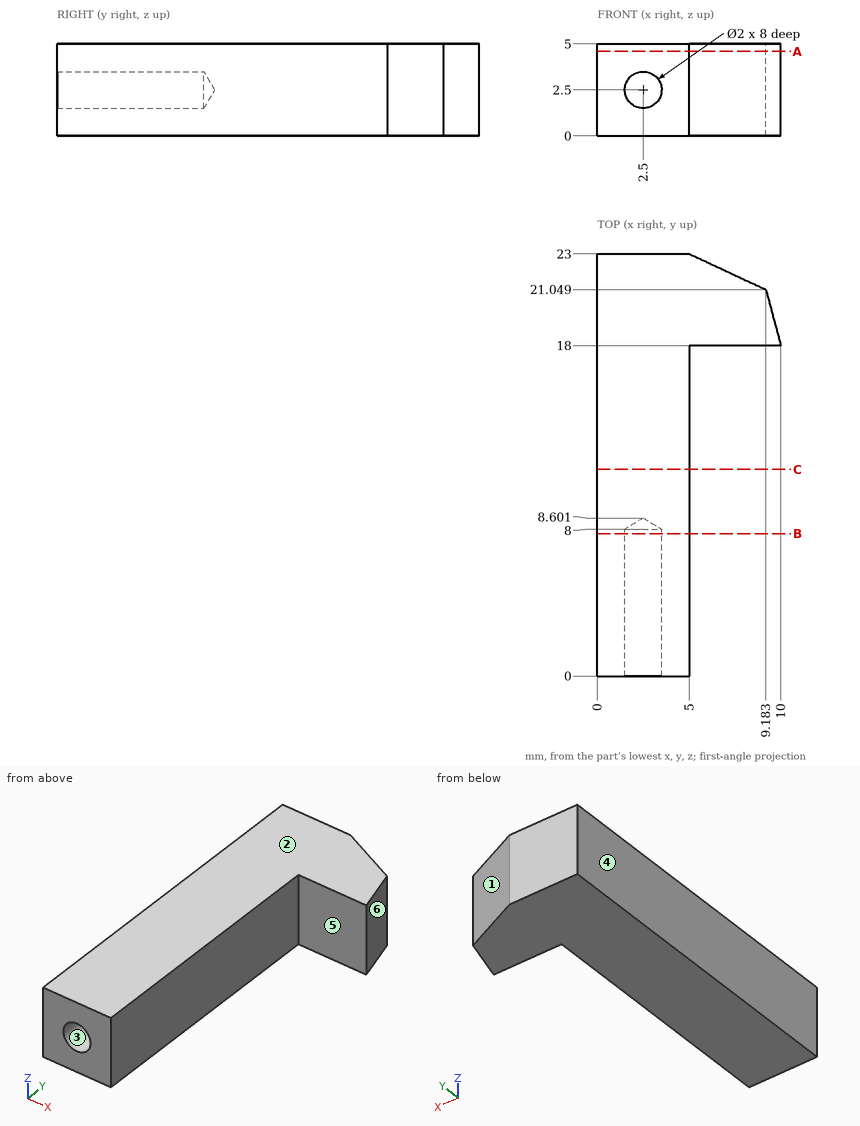
For this review, use the dimensioned drawing (mm, ordinates from the lowest corner) and the shaded views. A direction names the side the tool comes from. Give positions to 0.01 mm unless a question says otherwise; leave off trailing zeros. Write each loop counter-clockwise with the first axis right and the second up, starting at its lowest first coordinate (ties: lowest second). Pieces come first, ordered by that corner, then holes. Notation, with made-up numbers: M 11,48 L 35,48 A21 cw 35,79 Z; hole C 29,-3 d7. An arc over 180 degrees is marked long. Answer as a JSON object with one key per item and string values. Group by question number.
Item 1: Draft analysis for pull direction X (two halves, no side actions). For the marked faces 1, 2, 3 and 4, state which applies: +X half, -X half, draft (parallel to the pull), parting line (faces both ways), or undercut.
Item 2: For pin 1 Ø1.5 at (x, y) = (7.5, 10.5) entering from -Z; pin 2 Ø2.5 at (y, z) = (10.5, 3.5) entering from +X, all flat-tipped, find the tip position at first contact; note any pin that passes through.
Item 3: Consider section C-C on y = 11.25. Write out the cut boundary in (x, z), plus the area to 3 significant figures.
Item 4: For probe 1 along Z at (x, y) = (2.5, 5.25); probe 2 along X at (y, z) = (12.5, 1.3), list the stretches that pass through material, from the lowest coordinate up. Write a range as [from, to].
Item 5: Consider section B-B on y = 7.75. Write out the cut boundary in (x, z).
Item 6: Consider section A-A on z = 4.6. Write out the cut boundary in (x, y), plus the area to 3 significant figures.
Item 7: Tool access review of the marked faces 5 and 6: name each direction out of +Z, -Z, +X, -X, +Y, -Y from which nothing blocks a thin tool from reaching the whole face with its end or side.
Check result:
{
 "1": {"face 1": "+X half", "face 2": "draft", "face 3": "undercut", "face 4": "-X half"},
 "2": {"pin 1": "passes through", "pin 2": "stops at x = 5"},
 "3": {"outline": "M 0,0 L 5,0 L 5,5 L 0,5 Z", "area": "25.0 mm^2"},
 "4": {"probe 1": "z = [0, 1.5], [3.5, 5]", "probe 2": "x = [0, 5]"},
 "5": {"outline": "M 0,0 L 5,0 L 5,5 L 0,5 Z; hole C 2.5,2.5 d2"},
 "6": {"outline": "M 0,0 L 5,0 L 5,18 L 10,18 L 9.18,21.05 L 5,23 L 0,23 Z", "area": "133 mm^2"},
 "7": {"face 5": "+Z, -Z, +X, -Y", "face 6": "+Z, -Z, +X, +Y"}
}
